Print and shaded views of the part. All mm, measured from the part's lowest x, y and z. Give positions to 0.01 mm unless a question says otherwise; leave off trailing zeros. Loops run counter-clockwise (first coordinate to the right, second up) from the corner with the lowest first, then second, coordinate; pieces in that order, holes last. Notation, with made-up numbers: (30, 74.5) - (42, 74.5) arc R26 ccw to (42, 92.5) - close; hole circle Ø5 at (-25.75, 41.25). An arc over 180 degrees is marked (long way). Return JSON: item names as keys, results as strings.
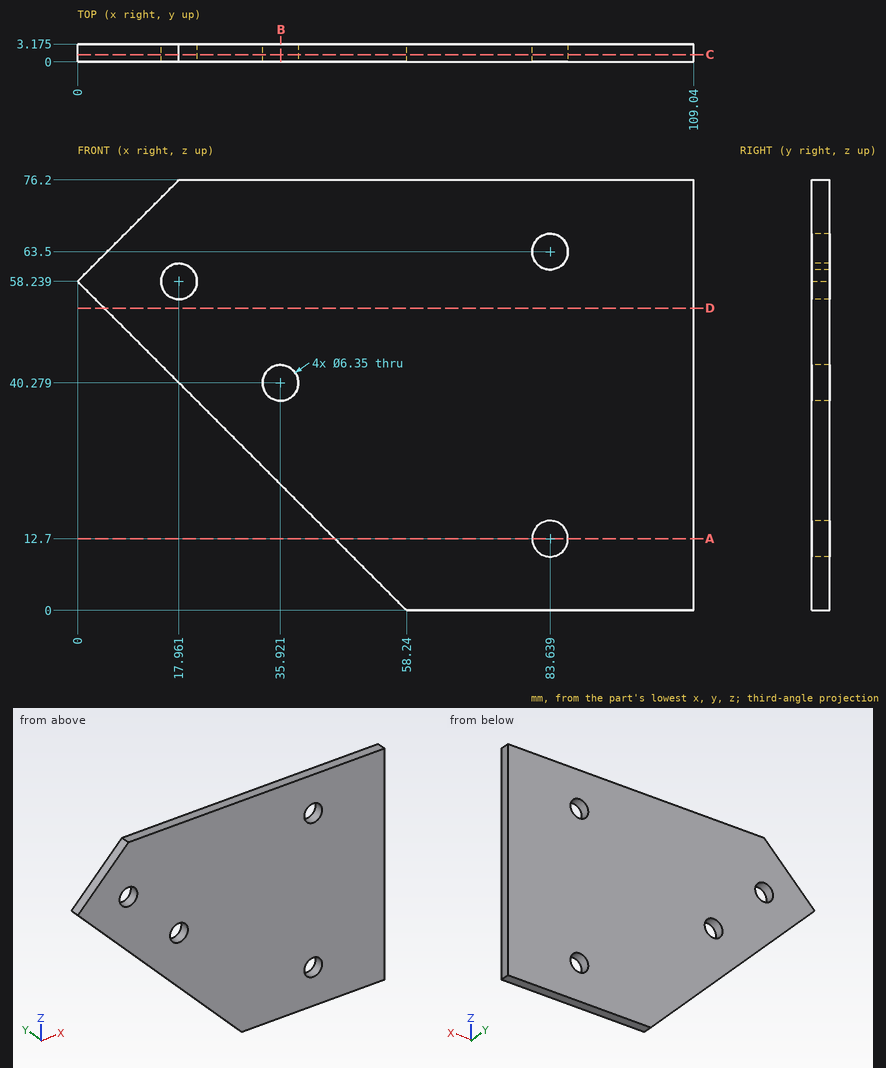
1. Drop a flat-ended pin along its axis: P1, Ø5, axis at x = 17.96, z = 58.24, coming from the +Y side. Give the stop position or say it passes through.
Values follow:
{"P1": "passes through"}
2. Cut at B-B, the plane x = 36. Write the cut outline in (y, z) (1 decimal).
Values follow:
{"outline": "(0, 22.2) - (3.2, 22.2) - (3.2, 37.1) - (0, 37.1) - close; (0, 43.5) - (3.2, 43.5) - (3.2, 76.2) - (0, 76.2) - close"}
3. Cut at C-C, the plane y = 1.3. Give the number of separate pieces and of enclosed holes in the cut face.
Values follow:
{"separate pieces": "1", "enclosed holes": "4"}
4. Cut at A-A, the plane z = 12.7. Write the cut outline in (x, y) (1 decimal).
Values follow:
{"outline": "(45.5, 0) - (80.5, 0) - (80.5, 3.2) - (45.5, 3.2) - close; (86.8, 0) - (109, 0) - (109, 3.2) - (86.8, 3.2) - close"}
5. Cut at D-D, the plane z = 53.5. Write the cut outline in (x, y) (1 decimal), plus the area to 3 significant figures.
Values follow:
{"outline": "(4.7, 0) - (109, 0) - (109, 3.2) - (4.7, 3.2) - close", "area": "331 mm²"}
6. Drill centre lines: probe 1 along X at (y, z) = (2.2, 43) (1 decimal); probe 2 along X at (y, z) = (2.6, 38); probe 3 along Z at (x, y) = (86, 2) (1 decimal). Where is each one in solid material? Low to high.
Values follow:
{"probe 1": "x = 15.2 to 34.3, 37.6 to 109", "probe 2": "x = 20.24 to 33.71, 38.13 to 109.04", "probe 3": "z = 0 to 10.6, 14.8 to 61.4, 65.6 to 76.2"}
